```python
from build123d import *

# Parameters (mm, degrees)
F0_W         = 2
F0_H         = 2
F0_W_2       = 11
F0_H_2       = 28
F0_W_3       = 35
F1_DEPTH     = 60
F2_ANGLE     = -90
F4_R         = 5
F4_2_R       = 5
F6_DEPTH     = 23.9
F7_R         = 1.99999
F8_T1_DEPTH  = 60
F8_T3_DEPTH  = 23
F8_T5_DEPTH  = 1e-05
F8_T7_DEPTH  = 1e-05
F8_T9_DEPTH  = 50
F8_T12_ANGLE = 90
F8_T14_ANGLE = 90
F8_T16_ANGLE = 90
F8_T18_ANGLE = 90
F8_T20_ANGLE = 90
F8_T21_DEPTH = 50
F8_T23_DEPTH = 22
F8_T25_DEPTH = 10
F8_T28_ANGLE = 90
F8_T30_ANGLE = 90
F8_T32_ANGLE = 90
F8_T34_ANGLE = 90


# Not quite as in the source:
# - a fillet or chamfer that OpenCascade refuses, or shapes differently, is made with other operations: its cross-section is extruded or revolved along the edge and cut away or added
# - a fillet or chamfer is up to 0.001 mm smaller than in the source, because OpenCascade refuses the exact size


with BuildPart() as f1:
    # F0 (on Front) → F1 (new body)
    with BuildSketch(Plane.XZ):
        with Locations((1, 1)):
            Rectangle(F0_W, F0_H)
        with Locations((7.5, 1)):
            Rectangle(F0_W_2, F0_H)
        with Locations((1, 16)):
            Rectangle(F0_W, F0_H_2)
        with Locations((14, 1)):
            Rectangle(F0_W, F0_H)
        with Locations((32.5, 1)):
            Rectangle(F0_W_3, F0_H)
        with Locations((14, 16)):
            Rectangle(F0_W, F0_H_2)
    extrude(amount=F1_DEPTH)


with BuildPart() as f2_1:
    # F2: copy of F1
    add(f1.part.rotate(Axis((15, 0, 16), (0, 0, 1)), F2_ANGLE))


with BuildPart() as f2_1_1:
    # F3: moved
    add(f2_1.part.moved(Location((58, 0, 0))))

    # F4#2
    f4_2_edges = [f2_1_1.edges().sort_by_distance(p)[0] for p in [
        (73, 1, 30),
        (73, 14, 30),
        (13, 14, 30),
        (13, 1, 30),
        (73, -35, 1),
    ]]
    fillet(f4_2_edges, radius=F4_2_R)


with BuildPart() as f1_1:
    add(f1.part)

    # F4
    f4_edges = [f1_1.edges().sort_by_distance(p)[0] for p in [
        (14, 0, 30),
        (1, 0, 30),
        (14, -60, 30),
        (1, -60, 30),
        (50, -60, 1),
    ]]
    fillet(f4_edges, radius=F4_R)

    add(f2_1_1.part)  # F6 merges F2_1
    # F5 (on face) → F6 (join)
    with BuildSketch(Plane.XY.offset(2)):
        Polygon((16.8020091951, 0), (15, 0), (15, -2), (17, -2), (17, 0), align=None)
    extrude(amount=F6_DEPTH)

    # F7 (radius 2 in the source; OpenCascade refuses exactly that, so slightly less here)
    f7_edges = [f1_1.edges().sort_by_distance(p)[0] for p in [
        (17, -2, 13.95),
    ]]
    fillet(f7_edges, radius=F7_R)

    # F8: fillet of radius 1 on 19 edges, made by hand

    # F8_s2 → F8_t1 (join)
    with BuildSketch(Plane.XZ):
        with BuildLine():
            ThreePointArc((2, 3), (2.2928932188, 2.2928932188), (3, 2))
            Line((3, 2), (2, 2))
            Line((2, 2), (2, 3))
        make_face()
    extrude(amount=F8_T1_DEPTH)

    # F8_s4 → F8_t3 (cut)
    with BuildSketch(Plane.XY.offset(2)):
        with BuildLine():
            ThreePointArc((13, 1), (13.2928932188, 1.7071067812), (14, 2))
            Line((14, 2), (13, 2))
            Line((13, 2), (13, 1))
        make_face()
        with BuildLine():
            ThreePointArc((73, 14), (72.7071067812, 13.2928932188), (72, 13))
            Line((72, 13), (73, 13))
            Line((73, 13), (73, 14))
        make_face()
        with BuildLine():
            ThreePointArc((73, 1), (72.7071067812, 1.7071067812), (72, 2))
            Line((72, 2), (73, 2))
            Line((73, 2), (73, 1))
        make_face()
        with BuildLine():
            ThreePointArc((13, 14), (13.2928932188, 13.2928932188), (14, 13))
            Line((14, 13), (13, 13))
            Line((13, 13), (13, 14))
        make_face()
    extrude(amount=F8_T3_DEPTH, mode=Mode.SUBTRACT)

    # F8_s6 → F8_t5 (cut)
    with BuildSketch(Plane.YZ.offset(15)):
        with BuildLine():
            ThreePointArc((-2, 24.9), (-1.7071067812, 25.6071067812), (-1, 25.9))
            Line((-1, 25.9), (-2, 25.9))
            Line((-2, 25.9), (-2, 24.9))
        make_face()
    extrude(amount=F8_T5_DEPTH, mode=Mode.SUBTRACT)

    # F8_s8 → F8_t7 (cut)
    with BuildSketch(Plane.XZ):
        with BuildLine():
            ThreePointArc((17, 24.9), (16.7071067812, 25.6071067812), (16, 25.9))
            Line((16, 25.9), (17, 25.9))
            Line((17, 25.9), (17, 24.9))
        make_face()
    extrude(amount=F8_T7_DEPTH, mode=Mode.SUBTRACT)

    # F8_s10 → F8_t9 (cut)
    with BuildSketch(Plane.YZ.offset(18)):
        with BuildLine():
            ThreePointArc((13, 29), (13.2928932188, 29.7071067812), (14, 30))
            Line((14, 30), (13, 30))
            Line((13, 30), (13, 29))
        make_face()
        with BuildLine():
            ThreePointArc((1, 30), (1.7071067812, 29.7071067812), (2, 29))
            Line((2, 29), (2, 30))
            Line((2, 30), (1, 30))
        make_face()
    extrude(amount=F8_T9_DEPTH, mode=Mode.SUBTRACT)

    # F8_s11 → F8_t12 (revolve, cut)
    with BuildSketch(Plane.XZ.offset(1e-05)):
        with BuildLine():
            ThreePointArc((17, 24.9), (16.7071067812, 25.6071067812), (16, 25.9))
            Line((16, 25.9), (17, 25.9))
            Line((17, 25.9), (17, 24.9))
        make_face()
    revolve(axis=Axis((15.00001, -1e-05, 25.9), (0, 0, -1)), revolution_arc=F8_T12_ANGLE, mode=Mode.SUBTRACT)

    # F8_s13 → F8_t14 (revolve, cut)
    with BuildSketch(Plane.YZ.offset(68)):
        with BuildLine():
            ThreePointArc((1, 30), (1.7071067812, 29.7071067812), (2, 29))
            Line((2, 29), (2, 30))
            Line((2, 30), (1, 30))
        make_face()
    revolve(axis=Axis((68, 2, 25), (0, 1, 0)), revolution_arc=F8_T14_ANGLE, mode=Mode.SUBTRACT)

    # F8_s15 → F8_t16 (revolve, cut)
    with BuildSketch(Plane.YZ.offset(18)):
        with BuildLine():
            ThreePointArc((1, 30), (1.7071067812, 29.7071067812), (2, 29))
            Line((2, 29), (2, 30))
            Line((2, 30), (1, 30))
        make_face()
    revolve(axis=Axis((18, 2, 25), (0, -1, 0)), revolution_arc=F8_T16_ANGLE, mode=Mode.SUBTRACT)

    # F8_s17 → F8_t18 (revolve, cut)
    with BuildSketch(Plane.YZ.offset(68)):
        with BuildLine():
            ThreePointArc((14, 30), (13.2928932188, 29.7071067812), (13, 29))
            Line((13, 29), (13, 30))
            Line((13, 30), (14, 30))
        make_face()
    revolve(axis=Axis((68, 13, 25), (0, 1, 0)), revolution_arc=F8_T18_ANGLE, mode=Mode.SUBTRACT)

    # F8_s19 → F8_t20 (revolve, cut)
    with BuildSketch(Plane.YZ.offset(18)):
        with BuildLine():
            ThreePointArc((13, 29), (13.2928932188, 29.7071067812), (14, 30))
            Line((14, 30), (13, 30))
            Line((13, 30), (13, 29))
        make_face()
    revolve(axis=Axis((18, 13, 25), (0, -1, 0)), revolution_arc=F8_T20_ANGLE, mode=Mode.SUBTRACT)

    # F8_s22 → F8_t21 (cut)
    with BuildSketch(Plane.XZ.offset(5)):
        with BuildLine():
            ThreePointArc((2, 29), (1.7071067812, 29.7071067812), (1, 30))
            Line((1, 30), (2, 30))
            Line((2, 30), (2, 29))
        make_face()
    extrude(amount=F8_T21_DEPTH, mode=Mode.SUBTRACT)

    # F8_s24 → F8_t23 (cut)
    with BuildSketch(Plane.XY.offset(3)):
        with BuildLine():
            ThreePointArc((2, -1), (1.7071067812, -0.2928932188), (1, 0))
            Line((1, 0), (2, 0))
            Line((2, 0), (2, -1))
        make_face()
        with BuildLine():
            ThreePointArc((2, -59), (1.7071067812, -59.7071067812), (1, -60))
            Line((1, -60), (2, -60))
            Line((2, -60), (2, -59))
        make_face()
    extrude(amount=F8_T23_DEPTH, mode=Mode.SUBTRACT)

    # F8_s26 → F8_t25 (cut)
    with BuildSketch(Plane.YZ.offset(3)):
        with BuildLine():
            ThreePointArc((-59, 2), (-59.7071067812, 1.7071067812), (-60, 1))
            Line((-60, 1), (-60, 2))
            Line((-60, 2), (-59, 2))
        make_face()
        with BuildLine():
            ThreePointArc((-1, 2), (-0.2928932188, 1.7071067812), (0, 1))
            Line((0, 1), (0, 2))
            Line((0, 2), (-1, 2))
        make_face()
    extrude(amount=F8_T25_DEPTH, mode=Mode.SUBTRACT)

    # F8_s27 → F8_t28 (revolve, cut)
    with BuildSketch(Plane.XZ.offset(5)):
        with BuildLine():
            ThreePointArc((2, 29), (1.7071067812, 29.7071067812), (1, 30))
            Line((1, 30), (2, 30))
            Line((2, 30), (2, 29))
        make_face()
    revolve(axis=Axis((2, -5, 25), (-1, 0, 0)), revolution_arc=F8_T28_ANGLE, mode=Mode.SUBTRACT)

    # F8_s29 → F8_t30 (revolve, cut)
    with BuildSketch(Plane.XZ.offset(55)):
        with BuildLine():
            ThreePointArc((1, 30), (1.7071067812, 29.7071067812), (2, 29))
            Line((2, 29), (2, 30))
            Line((2, 30), (1, 30))
        make_face()
    revolve(axis=Axis((2, -55, 25), (1, 0, 0)), revolution_arc=F8_T30_ANGLE, mode=Mode.SUBTRACT)

    # F8_s31 → F8_t32 (revolve, cut)
    with BuildSketch(Plane.XY.offset(3)):
        with BuildLine():
            ThreePointArc((2, -1), (1.7071067812, -0.2928932188), (1, 0))
            Line((1, 0), (2, 0))
            Line((2, 0), (2, -1))
        make_face()
    revolve(axis=Axis((3, 0, 3), (0, -1, 0)), revolution_arc=F8_T32_ANGLE, mode=Mode.SUBTRACT)

    # F8_s33 → F8_t34 (revolve, cut)
    with BuildSketch(Plane.XY.offset(3)):
        with BuildLine():
            ThreePointArc((2, -59), (1.7071067812, -59.7071067812), (1, -60))
            Line((1, -60), (2, -60))
            Line((2, -60), (2, -59))
        make_face()
    revolve(axis=Axis((3, -60, 3), (0, -1, 0)), revolution_arc=F8_T34_ANGLE, mode=Mode.SUBTRACT)


solid = f1_1.part
```
Input: part model. Units: mm. Frame: model coordinates. A direction names the side the tool comes from. Round coordinates to 2 decimals unless told otherwise and drop trailing zeros. Loops run counter-clockwise (first coordinate to the right, second up) from the corner with the lowest first, then second, coordinate; pieces in that order, holes last. Notation, with made-up numbers: (87, -24.5) - (145, -24.5) arc R24 ccw to (145, 12.5) - close; hole circle Ø8 at (-14, -24). An arc over 180 degrees is marked (long way). One line per item, written item: value. Start each with the question number.
(1) Access query for faces 5 (the flat face through (37, -22, 0)), 6 (the cylindrical face through (14.5, 14.49, 28.57)), 7 (the flat face through (43, 2, 15)), 8 (the flat face through (8, -30, 2)), 9 (the flat face through (50, -45, 1)). Directions: +Z, -Z, +X, -X, +Y, -Y. A direction counts if a zero-diameter tool reaches every point of the face in a straight line with its end or side. Return the directions, or none.
(2) Section D-D, the plane y = -22. Return loops of the section in (x, z), plus the area to 3 significant figures.
(3) Section B-B, the plane y = -49. Return loops of the section in (x, z), plus the area to 3 significant figures.
(4) Section C-C, the plane x = 9.5. Return loops of the section in (y, z).
(5) Section A-A, the plane z = 22. Count the separate pieces of the cut face and the enclosed holes in it, plus the area to 3 significant figures.
(6) Ray query, line 1 (Y direction, x = 42.5, z = 4); line 2 (Z direction, x = 41.5, y = -31.5). Return the intervals inside material, ascending. Write a range as [from, to].
(7) Contact query for flat-ended pins moving along their axis: P1, Ø6, axis at y = -35, z = 25.5, coming from the +X side; P2, Ø12, axis at x = 44, y = -40.5, coming from the +Z side; P3, Ø8, axis at x = 58.5, z = 15, coming from the -Y side. Output: stop coordinate, or through.
(8) Draft query along X for faces 1 (the cylindrical face through (14.5, 0.49, 28.57)), 2 (the flat face through (14, -30, 30)), 3 (the cylindrical face through (16.4, -1.43, 13.61)), 4 (the flat face through (2, -30, 16)). Return one class per face: +X half, -X half, draft (parallel to the pull), parting line (faces both ways), or undercut.
Results below:
1. face 5: -Z, +X, -X, +Y, -Y
1. face 6: +Z, -X, +Y
1. face 7: +Z, +X, -X
1. face 8: +Z, +Y, -Y
1. face 9: +Z, -Z, +X, -Y
2. outline: (0, 0) - (73, 0) - (73, 2) - (15, 2) - (15, 30) - (13, 30) - (13, 2) - (3, 2) arc R1 cw to (2, 3) - (2, 29) arc R1 ccw to (1, 30) - (0, 30) - close
2. area: 258 mm^2
3. outline: (0, 0) - (50, 0) - (50, 2) - (15, 2) - (15, 30) - (13, 30) - (13, 2) - (3, 2) arc R1 cw to (2, 3) - (2, 29) arc R1 ccw to (1, 30) - (0, 30) - close
3. area: 212 mm^2
4. outline: (-60, 0) - (0, 0) - (0, 1) arc R1 ccw to (-1, 2) - (-59, 2) arc R1 ccw to (-60, 1) - close
5. separate pieces: 3
5. enclosed holes: 0
5. area: 482 mm^2
6. line 1: [0, 2], [13, 15]
6. line 2: [0, 2]
7. P1: x = 15
7. P2: z = 2
7. P3: y = 0
8. face 1: -X half
8. face 2: draft
8. face 3: +X half
8. face 4: undercut
